Geometry: final body of the model. Coordinates: model frame, mm. Coordinates: 2 decimals unless noted, no trailing zeros. Order: outer loops, then holes, each group sorted by start corner. A loop starts at its lowest first (then second) coordinate and runs counter-clockwise, first axis right, second up. Notation, with made-up numbers: M 77,5 L 117,5 A23 ccw 117,29 Z; hole C 67,77 d2. An arc over 180 degrees is marked long. Use CSV: the item, a comma, the result in double quotes. Start each with the question number.
Q1. Section query D-D, the plane z = -56. Output: boundary loops of the cut face in (x, y) (3 decimals).
Q2. Section query C-C, the plane y = 1.6. State how many separate pieces and enclosed holes the cut face has, and give its area (3 significant figures).
Q3. Section query B-B, the plane x = -117.65. Output: boundary loops of the cut face in (y, z) (3 decimals).
Q4. First-contact query: P1, Ø1.6, axis at x = 54.5, y = 1, coming from the -Z side. Flat tip, straight axial feed; report the tip coordinate or a pass-through.
Q5. Section query A-A, the plane z = -16. Output: boundary loops of the cut face in (x, y) (3 decimals), and give its area (3 significant figures).
Q6. Ray query, probe 1 along X at (y, z) = (1.85, -6.35); probe 2 along X at (y, z) = (1.1, -18.5) (3 decimals); probe 3 along Z at (x, y) = (-117.65, 2.2). Return the intervals inside material, ascending.
from build123d import *

# Parameters (mm, degrees)
SKETCH1_W           = 3.175
SKETCH1_H           = 25.4
SKETCH1_W_2         = 25.4
SKETCH1_H_2         = 3.175
SKETCH1_R           = 3.5
BOSS_EXTRUDE1_DEPTH = 3.175


with BuildPart() as part:
    # Sketch1 → Boss-Extrude1 (new body)
    with BuildSketch(Plane(origin=(0, 0, 0), x_dir=(1, 0, 0), z_dir=(0, 1, 0))):
        Polygon((-111.3, 63.5), (-139.7, 63.5), (-139.7, -15.7), (139.7, -15.7), (139.7, 63.5), (111.3, 63.5), (111.3, 12.7), (-111.3, 12.7), align=None)
        with Locations((135.1125, 25.4)):
            Rectangle(SKETCH1_W, SKETCH1_H, mode=Mode.SUBTRACT)
        with Locations((50.8, -11.1125)):
            Rectangle(SKETCH1_W_2, SKETCH1_H_2, mode=Mode.SUBTRACT)
        with Locations((0, -11.1125)):
            Rectangle(SKETCH1_W_2, SKETCH1_H_2, mode=Mode.SUBTRACT)
        with Locations((-50.8, -11.1125)):
            Rectangle(SKETCH1_W_2, SKETCH1_H_2, mode=Mode.SUBTRACT)
        with Locations((-135.1125, 25.4)):
            Rectangle(SKETCH1_W, SKETCH1_H, mode=Mode.SUBTRACT)
        with Locations((-117.65, 6.35)):
            Circle(SKETCH1_R, mode=Mode.SUBTRACT)
        with Locations((117.65, 6.35)):
            Circle(SKETCH1_R, mode=Mode.SUBTRACT)
    extrude(amount=BOSS_EXTRUDE1_DEPTH)


solid = part.part
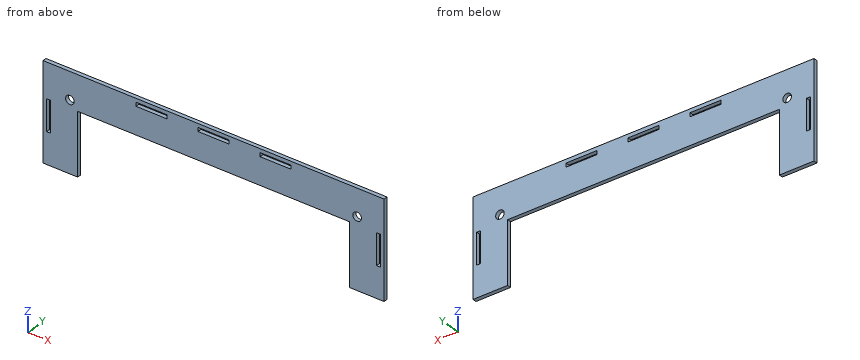
Responses:
1,outline,"M -139.7,0 L -111.3,0 L -111.3,3.175 L -139.7,3.175 Z; M 111.3,0 L 139.7,0 L 139.7,3.175 L 111.3,3.175 Z"
2,separate pieces,"1"
2,enclosed holes,"7"
2,area,"10,300 mm²"
3,outline,"M 0,-63.5 L 3.175,-63.5 L 3.175,-9.85 L 0,-9.85 Z; M 0,-2.85 L 3.175,-2.85 L 3.175,15.7 L 0,15.7 Z"
4,P1,"stops at z = -12.7"
5,outline,"M -139.7,0 L -136.7,0 L -136.7,3.175 L -139.7,3.175 Z; M -133.525,0 L -111.3,0 L -111.3,3.175 L -133.525,3.175 Z; M 111.3,0 L 133.525,0 L 133.525,3.175 L 111.3,3.175 Z; M 136.7,0 L 139.7,0 L 139.7,3.175 L 136.7,3.175 Z"
5,area,"160 mm²"
6,probe 1,"x = -139.7 to -121.15, -114.15 to 114.15, 121.15 to 139.7"
6,probe 2,"x = -139.7 to -136.7, -133.525 to -111.3, 111.3 to 133.525, 136.7 to 139.7"
6,probe 3,"z = -63.5 to -9.85, -2.85 to 15.7"
